```python
from build123d import *

# Parameters (mm, degrees)
F1_DEPTH  = 102.5
F2_T      = -2
F3_W      = 41
F3_H      = 98.5
F4_DEPTH  = 78.001
F5_W      = 98.5
F5_H      = 21.1715728753
F8_D      = 5
F9_W      = 28
F9_H      = 49
F10_DEPTH = 44.4274068712
F12_D     = 5
F12_DEPTH = 2.001
F14_D     = 3
F14_DEPTH = 12
F14_TIP   = 0.9012909285
F15_W     = 98.5
F15_H     = 2
F16_DEPTH = 20
F18_DEPTH = 25
F20_R     = 5.5
F21_DEPTH = 25
F22_R     = 5


with BuildPart() as f1:
    # F0 (on Front) → F1 (new body)
    with BuildSketch(Plane.XZ):
        Polygon((0, 80), (0, 0), (101, 0), (101, 20), (41, 80), align=None)
    extrude(amount=F1_DEPTH)

    # F2
    f2_openings = [f1.faces().sort_by_distance(p)[0] for p in [
        (0, -51.25, 40),
        (20.5, -51.25, 80),
    ]]
    offset(amount=F2_T, openings=f2_openings)

    # F3 (on face) → F4 (cut, through all)
    with BuildSketch(Plane.XY.offset(2)):
        with Locations((20.5, -51.25)):
            Rectangle(F3_W, F3_H)
    extrude(amount=F4_DEPTH, mode=Mode.SUBTRACT)

    # F5 (on face) → F6 (join, up to the last surface of F1)
    with BuildSketch(Plane(origin=(41, 0, 0), x_dir=(0, -1, 0), z_dir=(-1, 0, 0))):
        with Locations((51.25, 66.5857864376)):
            Rectangle(F5_W, F5_H)
    extrude(until=Until.LAST, dir=(1, 0, 0))

    # F8 (through all)
    with Locations(Plane(origin=(41, 0, 0), x_dir=(0, -1, 0), z_dir=(-1, 0, 0))):
        with Locations((85, 72), (14, 72)):
            Hole(F8_D / 2)

    # F9 (on face) → F10 (cut, through all)
    with BuildSketch(Plane(origin=(59.0857864376, 0, 59.0857864376), x_dir=(0.7071067812, 0, -0.7071067812), z_dir=(-0.7071067812, 0, -0.7071067812))):
        with Locations((30.405591591, 51.25)):
            Rectangle(F9_W, F9_H)
    extrude(amount=-F10_DEPTH, mode=Mode.SUBTRACT)

    # F12 (through all, one way)
    with BuildSketch(Plane(origin=(0, -100.5, 0), x_dir=(-1, 0, 0), z_dir=(0, 1, 0))):
        with Locations((-22, 72)):
            Circle(F12_D / 2)
    extrude(amount=-F12_DEPTH, mode=Mode.SUBTRACT)

    # F14
    with Locations(Plane(origin=(60.5, 0, 60.5), x_dir=(0.7071067812, 0, -0.7071067812), z_dir=(0.7071067812, 0, 0.7071067812))):
        with Locations((10.405591591, -51.75), (50.405591591, -51.75)):
            Hole(F14_D / 2, depth=F14_DEPTH)
            with Locations((0, 0, -(F14_DEPTH + F14_TIP / 2))):  # 118° drill point
                Cone(0, F14_D / 2, F14_TIP, mode=Mode.SUBTRACT)

    # F15 (on face) → F16 (cut)
    with BuildSketch(Plane(origin=(0, 0, 0), x_dir=(0, -1, 0), z_dir=(-1, 0, 0))):
        with Locations((51.25, 1)):
            Rectangle(F15_W, F15_H)
    extrude(amount=-F16_DEPTH, mode=Mode.SUBTRACT)

    # F17 (on face) → F18 (cut)
    with BuildSketch(Plane.XZ.offset(102.5)):
        Polygon((0, 35), (0, 0), (35, 0), (35, 15), (15, 35), align=None)
    extrude(amount=-F18_DEPTH, mode=Mode.SUBTRACT)

    # F20 (on offset) → F21 (cut)
    with BuildSketch(Plane(origin=(44, 0, 0), x_dir=(0, -1, 0), z_dir=(-1, 0, 0))):
        with Locations((85, 72)):
            Circle(F20_R)
        with Locations((14, 72)):
            Circle(F20_R)
    extrude(amount=-F21_DEPTH, mode=Mode.SUBTRACT)

    # F22
    f22_edges = [f1.edges().sort_by_distance(p)[0] for p in [
        (35, -77.5, 1),
        (35, -101.5, 15),
        (15, -101.5, 35),
        (20, -77.5, 1),
        (20, -2, 1),
        (0, -1, 80),
        (0, -101.5, 80),
        (0, -101.5, 35),
    ]]
    fillet(f22_edges, radius=F22_R)


solid = f1.part
```
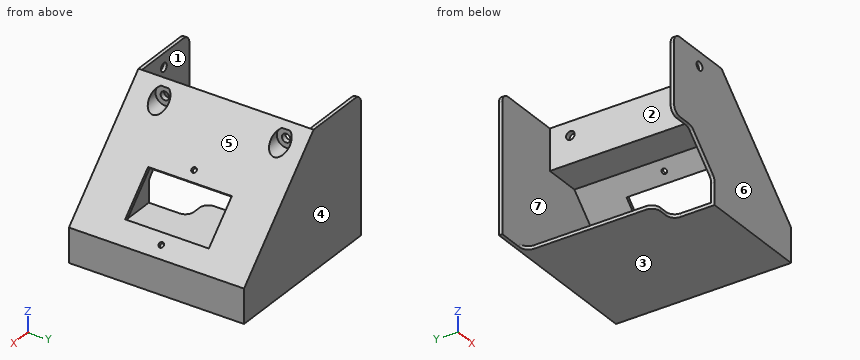
The listing builds one solid part. Answer for the finished solid, in the listing's coordinates (mm). Face numbers are marked on the shaded views. A direction names the side the tool comes from. Coordinates: 2 decimals unless noted, no trailing zeros. Write each loop counter-clockwise with the first axis right and the second up, starting at its lowest first coordinate (ties: lowest second). Pieces come first, ordered by that corner, then holes.
Q1. Section A-A, the plane z = 72 is taken. Write down the section's boundary in (x, y), then the cut area to 3 significant figures.
Returned:
outline: (0, -102.5) - (19.5, -102.5) - (19.5, -100.5) - (0, -100.5) - close; (0, -2) - (41, -2) - (41, -11.5) - (44, -11.5) - (44, -8.5) - (49, -8.5) - (49, 0) - (0, 0) - close; (24.5, -102.5) - (49, -102.5) - (49, -90.5) - (44, -90.5) - (44, -87.5) - (41, -87.5) - (41, -100.5) - (24.5, -100.5) - close; (41, -82.5) - (44, -82.5) - (44, -79.5) - (49, -79.5) - (49, -19.5) - (44, -19.5) - (44, -16.5) - (41, -16.5) - close
area: 834 mm2
Q2. Find the intervals of material crossed by line 1 along Y through (x, z) = (47.5, 72); line 2 along Z through (x, y) = (47.25, -85); line 3 along Y through (x, z) = (62, 52.5), in increasing order.
Returned:
line 1: y = -102.5 to -90.5, -79.5 to -19.5, -8.5 to 0
line 2: z = 0 to 2, 56 to 66.5
line 3: y = -102.5 to -100.5, -2 to 0
Q3. Section D-D, the plane z = 60 is taken. Write down the section's boundary in (x, y), then the cut area to 3 significant figures.
Returned:
outline: (0, -102.5) - (61, -102.5) - (61, 0) - (0, 0) - (0, -2) - (41, -2) - (41, -100.5) - (0, -100.5) - close
area: 2,210 mm2
Q4. Given P1, Ø19, axis at y = -55, z = 67, coming from the -X side; P2, Ø5, axis at y = -55.5, z = 10.5, coming from the -X side; P3, Ø1.5, axis at x = 32.5, z = 15, coming from the +Y side; P4, Ø6.5, axis at x = 86.5, z = 43, coming from the -Y side, each flat-ended and moving along its own axis, determine where each tip first touches the part or whether it passes through.
Returned:
P1: stops at x = 41
P2: stops at x = 99
P3: stops at y = 0
P4: passes through
Q5. Which of the six approach directions +Z, -Z, +X, -X, +Y, -Y give full straight-line access (tool end or side, diameter ignored) to the marked faces 1, 2 and 3?
Returned:
face 1: -X
face 2: +Z, -X
face 3: -Z, +X, -X, +Y, -Y
Q6. The mould has two halves that part along Y. Classify the marked faces 4, 5, 6 and 7: released by +Y, released by -Y, zero draft, split by the parting line, or undercut.
Returned:
face 4: released by +Y
face 5: zero draft
face 6: released by -Y
face 7: undercut
Q7. Section C-C, the plane y = -85 is taken. Write down the section's boundary in (x, z).
Returned:
outline: (35, 0) - (101, 0) - (101, 20) - (54.5, 66.5) - (44, 66.5) - (44, 69.5) - (41, 69.5) - (41, 56) - (62.17, 56) - (99, 19.17) - (99, 2) - (35, 2) - close; (41, 74.5) - (44, 74.5) - (44, 77) - (41, 80) - close
Q8. Section B-B, the plane x = 22 is taken. Write down the section's boundary in (y, z), then the cut area to 3 significant figures.
Returned:
outline: (-102.5, 28) - (-100.5, 28) - (-100.5, 69.5) - (-102.5, 69.5) - close; (-102.5, 74.5) - (-100.5, 74.5) - (-100.5, 80) - (-102.5, 80) - close; (-76.5, 0) - (0, 0) - (0, 80) - (-2, 80) - (-2, 2) - (-76.5, 2) - close
area: 403 mm2
